from build123d import *

# Parameters (mm, degrees)
SKETCH1_R           = 31.75
BOSS_EXTRUDE1_DEPTH = 25.4
SKETCH2_R           = 4.845598066
SKETCH2_R_2         = 2.7
BOSS_EXTRUDE2_DEPTH = 3.175
CUT_EXTRUDE1_REACH  = 53.588
SKETCH3_R           = 2.7


with BuildPart() as part:
    # Sketch1 → Boss-Extrude1 (new body)
    with BuildSketch(Plane.XY):
        Circle(SKETCH1_R)
    extrude(amount=BOSS_EXTRUDE1_DEPTH)

    # Sketch2 → Boss-Extrude2 (add)
    with BuildSketch(Plane.XY.offset(25.4)):
        Circle(SKETCH2_R)
        Circle(SKETCH2_R_2, mode=Mode.SUBTRACT)
    extrude(amount=BOSS_EXTRUDE2_DEPTH)

    # Sketch3 → Cut-Extrude1 (cut, up to next)
    with BuildSketch(Plane.XY.offset(25.4), mode=Mode.PRIVATE) as cut_extrude1_sk1:
        Circle(SKETCH3_R)
    cut_extrude1_tool1 = extrude(cut_extrude1_sk1.sketch, amount=-CUT_EXTRUDE1_REACH, mode=Mode.PRIVATE) & part.part
    add(cut_extrude1_tool1.solids().sort_by_distance((0, 0, 25.4))[0], mode=Mode.SUBTRACT)


solid = part.part
Can you work these out from the model? Positions are in its coordinate system, mm. A direction names the side the tool comes from. Coordinates: 2 decimals unless noted, no trailing zeros. Loops run counter-clockwise (first coordinate to the right, second up) from the corner with the lowest first, then second, coordinate; pieces in that order, holes last. Notation, with made-up numbers: (-12.75, 21) - (16.25, 21) arc R23 ccw to (16.25, 31) - close; hole circle Ø2 at (8, 2). An arc over 180 degrees is marked (long way). Put each result on its own line as item: value. Start each with the question number.
Item 1: If I drill on line 1 along Y through (x, z) = (0, 26.2); line 2 along Z through (x, y) = (5, 26); line 3 along Y through (x, z) = (0, 7.5), over which ranges is the centre line in solid material (lowest first)?
Item 2: Suppose I cut it at A-A (y = 0). Please give me the cut outline in (x, z) (3 decimals).
Item 3: For pin 1 (1 mm diameter, centred on x = 7.5, z = 15, fed in from +Y); pin 2 (2 mm diameter, centred on y = 10.5, z = 18.5, fed in from -X); pin 3 (1.5 mm diameter, centred on x = -12.5, y = -1.5, fed in from +Z); pin 4 (3 mm diameter, centred on x = 0, y = 0, fed in from +Z), each with a flat end and sliding along its axis, tell me the tip position at first contact or that it passes through.
Item 4: Suppose I cut it at C-C (z = 2.75). Please give me the cut outline in (x, y).
Item 5: Suppose I cut it at D-D (x = 26). Please give me the cut outline in (y, z), and give its area (3 significant figures).
Item 6: Which directions (+Z, -Z, +X, -X, +Y, -Y) give clear straight access to the entire face, cutting with the end or side of a thin tool? Please do faces 1 (the face through (4.62, 1.46, 26.97)), 2 (the face through (7, 0, 0)).
Here are the results:
1. line 1: -4.85 to -2.7, 2.7 to 4.85
1. line 2: 0 to 25.4
1. line 3: -31.75 to -2.7, 2.7 to 31.75
2. outline: (-31.75, 0) - (-2.7, 0) - (-2.7, 28.575) - (-4.846, 28.575) - (-4.846, 25.4) - (-31.75, 25.4) - close; (2.7, 0) - (31.75, 0) - (31.75, 25.4) - (4.846, 25.4) - (4.846, 28.575) - (2.7, 28.575) - close
3. pin 1: y = 30.97
3. pin 2: x = -30.3
3. pin 3: z = 25.4
3. pin 4: through
4. outline: circle Ø63.5 at (0, 0); hole circle Ø5.4 at (0, 0)
5. outline: (-18.22, 0) - (18.22, 0) - (18.22, 25.4) - (-18.22, 25.4) - close
5. area: 926 mm²
6. face 1: +Z
6. face 2: -Z, +X, -X, +Y, -Y
